For this review, take the finished solid that the model builds, in its own axes (mm). Face numbers are marked on the shaded views. Give positions to 0.01 mm unless a question says otherwise; leave off trailing zeros. Write each loop counter-clockwise with the first axis right and the second up, starting at its lowest first coordinate (ties: lowest second). Pieces come first, ordered by that corner, then holes.
1) We need section A-A on z = 0. Give the boundary of the cut face in (x, y).
2) Wall thickness on line 1 along X through (y, z) = (27.5, 0); line 2 along X through (y, z) = (8.5, 40); line 3 along Z through (x, y) = (53.5, 11): over which ranges is each line inside the solid? List them lowest first.
3) For P1, Ø3, axis at y = 11, z = -8, coming from the -X side; P2, Ø12, axis at x = 12, z = -37, coming from the -Y side; P3, Ø3, axis at y = 18, z = 25.5, coming from the +X side; P4, Ø4, axis at x = 40.5, y = 31.5, coming from the +Z side, all flat-tipped, find the tip position at first contact; note any pin that passes through.
4) We need section B-B on x = 0. Give the boundary of the cut face in (y, z).
5) Draft analysis for pull direction X (two halves, no side actions). For the marked faces 1, 2 and 3, state which applies: pulls with the +X half, pulls with the -X half, needs draft (parallel to the pull), parting line crosses it, or undercut.
from build123d import *

# Parameters (mm, degrees)
SKETCH2_W           = 10
SKETCH2_H           = 45
BOSS_EXTRUDE1_DEPTH = 45


with BuildPart() as part:
    # Sketch2 → Revolve1 (revolve)
    with BuildSketch(Plane.XY):
        with Locations((55, 22.5)):
            Rectangle(SKETCH2_W, SKETCH2_H)
    revolve(axis=Axis((0, -1000, 0), (0, 1, 0)))

    # Sketch3 → Boss-Extrude1 (add)
    with BuildSketch(Plane(origin=(0, 0, 0), x_dir=(1, 0, 0), z_dir=(0, 1, 0))):
        with BuildLine():
            Line((4.502343049, 64.84388103), (3.76078814, 59.88202128))
            ThreePointArc((3.76078814, 59.88202128), (7.831571533, 59.486691682), (11.865965175, 58.81495448))
            Line((11.865965175, 58.81495448), (12.43390194, 63.799671493))
            ThreePointArc((12.43390194, 63.799671493), (8.484202494, 64.443915989), (4.502343049, 64.84388103))
        make_face()
        with BuildLine():
            Line((21.131760798, 61.469087235), (19.131249958, 56.868227289))
            ThreePointArc((19.131249958, 56.868227289), (22.961005942, 55.432771951), (26.684072572, 53.739745728))
            Line((26.684072572, 53.739745728), (28.522797059, 58.407619777))
            ThreePointArc((28.522797059, 58.407619777), (24.874423104, 60.052169613), (21.131760798, 61.469087235))
        make_face()
        with BuildLine():
            Line((36.321083972, 53.905276728), (33.197948708, 49.978957588))
            ThreePointArc((33.197948708, 49.978957588), (36.525685741, 47.601200417), (39.683704522, 45.002262115))
            Line((39.683704522, 45.002262115), (42.667910694, 49.035185296))
            ThreePointArc((42.667910694, 49.035185296), (39.569492886, 51.567967119), (36.321083972, 53.905276728))
        make_face()
        with BuildLine():
            Line((49.035185296, 42.667910694), (45.002262115, 39.683704522))
            ThreePointArc((45.002262115, 39.683704522), (47.601200417, 36.525685741), (49.978957588, 33.197948708))
            Line((49.978957588, 33.197948708), (53.905276728, 36.321083972))
            ThreePointArc((53.905276728, 36.321083972), (51.567967119, 39.569492886), (49.035185296, 42.667910694))
        make_face()
        with BuildLine():
            Line((58.407619777, 28.522797059), (53.739745728, 26.684072572))
            ThreePointArc((53.739745728, 26.684072572), (55.432771951, 22.961005942), (56.868227289, 19.131249958))
            Line((56.868227289, 19.131249958), (61.469087235, 21.131760798))
            ThreePointArc((61.469087235, 21.131760798), (60.052169613, 24.874423104), (58.407619777, 28.522797059))
        make_face()
        with BuildLine():
            Line((63.799671493, 12.43390194), (58.81495448, 11.865965175))
            ThreePointArc((58.81495448, 11.865965175), (59.486691682, 7.831571533), (59.88202128, 3.76078814))
            Line((59.88202128, 3.76078814), (64.84388103, 4.502343049))
            ThreePointArc((64.84388103, 4.502343049), (64.443915989, 8.484202494), (63.799671493, 12.43390194))
        make_face()
        with BuildLine():
            Line((64.84388103, -4.502343049), (59.88202128, -3.76078814))
            ThreePointArc((59.88202128, -3.76078814), (59.486691682, -7.831571533), (58.81495448, -11.865965175))
            Line((58.81495448, -11.865965175), (63.799671493, -12.43390194))
            ThreePointArc((63.799671493, -12.43390194), (64.443915989, -8.484202494), (64.84388103, -4.502343049))
        make_face()
        with BuildLine():
            Line((61.469087235, -21.131760798), (56.868227289, -19.131249958))
            ThreePointArc((56.868227289, -19.131249958), (55.432771951, -22.961005942), (53.739745728, -26.684072572))
            Line((53.739745728, -26.684072572), (58.407619777, -28.522797059))
            ThreePointArc((58.407619777, -28.522797059), (60.052169613, -24.874423104), (61.469087235, -21.131760798))
        make_face()
        with BuildLine():
            Line((53.905276728, -36.321083972), (49.978957588, -33.197948708))
            ThreePointArc((49.978957588, -33.197948708), (47.601200417, -36.525685741), (45.002262115, -39.683704522))
            Line((45.002262115, -39.683704522), (49.035185296, -42.667910694))
            ThreePointArc((49.035185296, -42.667910694), (51.567967119, -39.569492886), (53.905276728, -36.321083972))
        make_face()
        with BuildLine():
            Line((42.667910694, -49.035185296), (39.683704522, -45.002262115))
            ThreePointArc((39.683704522, -45.002262115), (36.525685741, -47.601200417), (33.197948708, -49.978957588))
            Line((33.197948708, -49.978957588), (36.321083972, -53.905276728))
            ThreePointArc((36.321083972, -53.905276728), (39.569492886, -51.567967119), (42.667910694, -49.035185296))
        make_face()
        with BuildLine():
            Line((28.522797059, -58.407619777), (26.684072572, -53.739745728))
            ThreePointArc((26.684072572, -53.739745728), (22.961005942, -55.432771951), (19.131249958, -56.868227289))
            Line((19.131249958, -56.868227289), (21.131760798, -61.469087235))
            ThreePointArc((21.131760798, -61.469087235), (24.874423104, -60.052169613), (28.522797059, -58.407619777))
        make_face()
        with BuildLine():
            Line((12.43390194, -63.799671493), (11.865965175, -58.81495448))
            ThreePointArc((11.865965175, -58.81495448), (7.831571533, -59.486691682), (3.76078814, -59.88202128))
            Line((3.76078814, -59.88202128), (4.502343049, -64.84388103))
            ThreePointArc((4.502343049, -64.84388103), (8.484202494, -64.443915989), (12.43390194, -63.799671493))
        make_face()
        with BuildLine():
            Line((-4.502343049, -64.84388103), (-3.76078814, -59.88202128))
            ThreePointArc((-3.76078814, -59.88202128), (-7.831571533, -59.486691682), (-11.865965175, -58.81495448))
            Line((-11.865965175, -58.81495448), (-12.43390194, -63.799671493))
            ThreePointArc((-12.43390194, -63.799671493), (-8.484202494, -64.443915989), (-4.502343049, -64.84388103))
        make_face()
        with BuildLine():
            Line((-21.131760798, -61.469087235), (-19.131249958, -56.868227289))
            ThreePointArc((-19.131249958, -56.868227289), (-22.961005942, -55.432771951), (-26.684072572, -53.739745728))
            Line((-26.684072572, -53.739745728), (-28.522797059, -58.407619777))
            ThreePointArc((-28.522797059, -58.407619777), (-24.874423104, -60.052169613), (-21.131760798, -61.469087235))
        make_face()
        with BuildLine():
            Line((-36.321083972, -53.905276728), (-33.197948708, -49.978957588))
            ThreePointArc((-33.197948708, -49.978957588), (-36.525685741, -47.601200417), (-39.683704522, -45.002262115))
            Line((-39.683704522, -45.002262115), (-42.667910694, -49.035185296))
            ThreePointArc((-42.667910694, -49.035185296), (-39.569492886, -51.567967119), (-36.321083972, -53.905276728))
        make_face()
        with BuildLine():
            Line((-49.035185296, -42.667910694), (-45.002262115, -39.683704522))
            ThreePointArc((-45.002262115, -39.683704522), (-47.601200417, -36.525685741), (-49.978957588, -33.197948708))
            Line((-49.978957588, -33.197948708), (-53.905276728, -36.321083972))
            ThreePointArc((-53.905276728, -36.321083972), (-51.567967119, -39.569492886), (-49.035185296, -42.667910694))
        make_face()
        with BuildLine():
            Line((-58.407619777, -28.522797059), (-53.739745728, -26.684072572))
            ThreePointArc((-53.739745728, -26.684072572), (-55.432771951, -22.961005942), (-56.868227289, -19.131249958))
            Line((-56.868227289, -19.131249958), (-61.469087235, -21.131760798))
            ThreePointArc((-61.469087235, -21.131760798), (-60.052169613, -24.874423104), (-58.407619777, -28.522797059))
        make_face()
        with BuildLine():
            Line((-63.799671493, -12.43390194), (-58.81495448, -11.865965175))
            ThreePointArc((-58.81495448, -11.865965175), (-59.486691682, -7.831571533), (-59.88202128, -3.76078814))
            Line((-59.88202128, -3.76078814), (-64.84388103, -4.502343049))
            ThreePointArc((-64.84388103, -4.502343049), (-64.443915989, -8.484202494), (-63.799671493, -12.43390194))
        make_face()
        with BuildLine():
            Line((-64.84388103, 4.502343049), (-59.88202128, 3.76078814))
            ThreePointArc((-59.88202128, 3.76078814), (-59.486691682, 7.831571533), (-58.81495448, 11.865965175))
            Line((-58.81495448, 11.865965175), (-63.799671493, 12.43390194))
            ThreePointArc((-63.799671493, 12.43390194), (-64.443915989, 8.484202494), (-64.84388103, 4.502343049))
        make_face()
        with BuildLine():
            Line((-61.469087235, 21.131760798), (-56.868227289, 19.131249958))
            ThreePointArc((-56.868227289, 19.131249958), (-55.432771951, 22.961005942), (-53.739745728, 26.684072572))
            Line((-53.739745728, 26.684072572), (-58.407619777, 28.522797059))
            ThreePointArc((-58.407619777, 28.522797059), (-60.052169613, 24.874423104), (-61.469087235, 21.131760798))
        make_face()
        with BuildLine():
            Line((-53.905276728, 36.321083972), (-49.978957588, 33.197948708))
            ThreePointArc((-49.978957588, 33.197948708), (-47.601200417, 36.525685741), (-45.002262115, 39.683704522))
            Line((-45.002262115, 39.683704522), (-49.035185296, 42.667910694))
            ThreePointArc((-49.035185296, 42.667910694), (-51.567967119, 39.569492886), (-53.905276728, 36.321083972))
        make_face()
        with BuildLine():
            Line((-42.667910694, 49.035185296), (-39.683704522, 45.002262115))
            ThreePointArc((-39.683704522, 45.002262115), (-36.525685741, 47.601200417), (-33.197948708, 49.978957588))
            Line((-33.197948708, 49.978957588), (-36.321083972, 53.905276728))
            ThreePointArc((-36.321083972, 53.905276728), (-39.569492886, 51.567967119), (-42.667910694, 49.035185296))
        make_face()
        with BuildLine():
            Line((-28.522797059, 58.407619777), (-26.684072572, 53.739745728))
            ThreePointArc((-26.684072572, 53.739745728), (-22.961005942, 55.432771951), (-19.131249958, 56.868227289))
            Line((-19.131249958, 56.868227289), (-21.131760798, 61.469087235))
            ThreePointArc((-21.131760798, 61.469087235), (-24.874423104, 60.052169613), (-28.522797059, 58.407619777))
        make_face()
        with BuildLine():
            Line((-12.43390194, 63.799671493), (-11.865965175, 58.81495448))
            ThreePointArc((-11.865965175, 58.81495448), (-7.831571533, 59.486691682), (-3.76078814, 59.88202128))
            Line((-3.76078814, 59.88202128), (-4.502343049, 64.84388103))
            ThreePointArc((-4.502343049, 64.84388103), (-8.484202494, 64.443915989), (-12.43390194, 63.799671493))
        make_face()
    extrude(amount=BOSS_EXTRUDE1_DEPTH)


solid = part.part
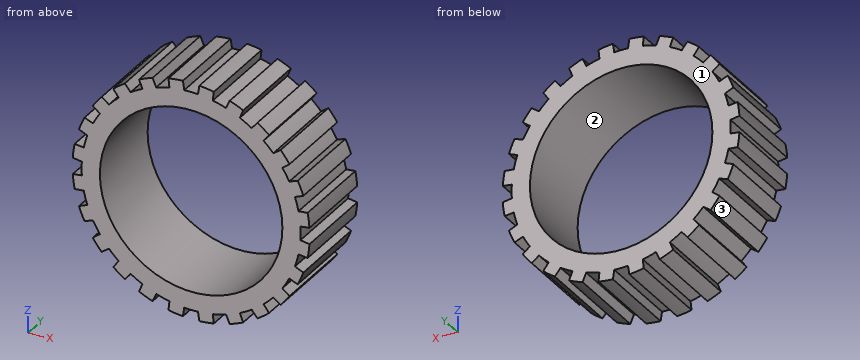
Results list:
1. outline: (-60, 0) - (-50, 0) - (-50, 45) - (-60, 45) - close; (50, 0) - (60, 0) - (60, 45) - (50, 45) - close
2. line 1: x = -60 to -50, 50 to 60
2. line 2: x = -51.23 to -45.43, -44.72 to -30, 30 to 44.72, 45.43 to 51.23
2. line 3: z = -36.92 to -36, -27.16 to 27.16, 36 to 36.92
3. P1: stops at x = -64.67
3. P2: passes through
3. P3: stops at x = 60.41
3. P4: stops at z = 52.37
4. outline: (0, -60) - (45, -60) - (45, -50) - (0, -50) - close; (0, 50) - (45, 50) - (45, 60) - (0, 60) - close
5. face 1: needs draft
5. face 2: undercut
5. face 3: pulls with the -X half
